Autodesk Inventor part; units mm, degrees
ref_plane "YZ Plane" through (0, 0, 0) normal (1, 0, 0) x (0, 1, 0)
ref_plane "XZ Plane" through (0, 0, 0) normal (0, 1, 0) x (-1, 0, 0)
ref_plane "XY Plane" through (0, 0, 0) normal (0, 0, 1) x (1, 0, 0)
sketch "Sketch1" plane through (0, 0, 0) normal (0, 1, 0) x (-1, 0, 0)
  line L0 (0, 0) -> (28.575, 0)
  line L1 (28.575, 0) -> (0, 0)
  line L2 (0, 0) -> (-14.2875, -24.7467)
  line L3 (0, 0) -> (28.575, 0) construction
  line L4 (0, 0) -> (-14.2875, 24.7467)
  line L5 (0, 0) -> (28.575, 0) construction
  circle A0 centre (28.575, 0) radius 2.54
  circle A1 centre (-14.2875, -24.7467) radius 2.54
  circle A2 centre (-14.2875, 24.7467) radius 2.54
  circle A3 centre (0, 0) radius 3.175
  circle A4 centre (0, 0) radius 6.35
  line L6 (-1.5875, -2.7496) -> (0, 0)
  line L7 (0, 0) -> (-6.35, 0)
  circle A5 centre (-14.2875, 24.7467) radius 3.81
  circle A6 centre (28.575, 0) radius 3.81
  circle A7 centre (-14.2875, -24.7467) radius 3.81
  line L8 (30.6811, 3.175) -> (-12.1814, 27.9217)
  line L9 (28.2054, -3.792) -> (-10.8187, -26.3226)
  line L10 (-18.0975, 24.7467) -> (-18.0975, -24.7467)
  line L11 (0, 0) -> (5.0525, -8.8146)
  line L12 (0, 0) -> (5.1463, 8.7602)
  line L13 (0, 0) -> (-10.16, 0)
  arc A8 (28.2054, -3.792) -> (-10.8187, -26.3226) centre (24.4473, -42.344) ccw
  arc A9 (-10.8187, 26.3226) -> (28.2054, 3.792) centre (24.4473, 42.344) ccw
  arc A10 (-17.3867, -22.5305) -> (-17.3867, 22.5305) centre (-48.8947, 0) ccw
  point P0 (5.1074, 8.7829)
  point P1 (-10.16, 0.0317)
  point P2 (30.2716, 3.4114)
  point P3 (28.2054, 3.792)
  point P4 (-10.8187, 26.3226)
  point P5 (-17.3867, 22.5305)
  point P6 (-17.3867, -22.5305)
  dimension "d9" = 6.35
  dimension "d41" = 12.7
  dimension "d0" = 28.575
  dimension "d1" = 28.575
  dimension "d2" = 120
  dimension "d3" = 28.575
  dimension "d4" = 120
  dimension "d5" = 5.08
  dimension "d6" = 5.08
  dimension "d7" = 5.08
  dimension "d42" = 7.62
  dimension "d43" = 7.62
  dimension "d44" = 7.62
  dimension "d47" = 10.16
  dimension "d48" = 10.16
  dimension "d49" = 10.16
  dimension "d52" = 360
extrude "Extrusion4" add sketch "Sketch1" along normal blind 12.7 contours A3 L12 A4 L0 | L0 A4 L11 A3 | A3 L11 A4 L2 | L2 A4 L7 A3 | A3 L7 A4 L4 | L4 A4 L12 A3 | A4 L12 A9 A6 L0 | L0 A6 A8 L11 A4 | A4 L11 A8 A7 L2 | L2 A7 A10 L13 A4 | A4 L13 A10 A5 L4 | L4 A5 A9 L12 A4 | A6 L8 | A7 | A5 picked at (31.8987, 0.5122)
sketch "Sketch11" plane through (0, 12.7, 0) normal (0, 1, 0) x (1, 0, 0)
  arc A0 (10.8187, -26.3226) -> (-28.2054, -3.792) centre (-24.4473, -42.344) ccw
  arc A1 (17.3867, 22.5305) -> (17.3867, -22.5305) centre (48.8947, 0) ccw
  arc A2 (10.8187, -26.3226) -> (17.3867, -22.5305) centre (14.2875, -24.7467) ccw
  line L0 (0, 0) -> (14.2875, -24.7467)
  circle A3 centre (14.2875, -24.7467) radius 2.54
  line L1 (14.2875, -24.7467) -> (8.2579, -14.3032)
  line L2 (14.2875, -24.7467) -> (7.9375, -13.7482)
  line L3 (7.9375, -13.7482) -> (11.895, -11.4633)
  line L4 (7.9375, -13.7482) -> (3.98, -16.033)
  circle A4 centre (14.2875, 24.7467) radius 2.54
  line L5 (0, 0) -> (14.2875, 24.7467)
  line L6 (14.2875, 24.7467) -> (7.9375, 13.7482)
  line L7 (7.9375, 13.7482) -> (0, 0)
  circle A5 centre (-28.575, 0) radius 2.54
  line L8 (0, 0) -> (-28.575, 0)
  line L9 (-28.575, 0) -> (-15.875, 0)
  line L10 (-15.875, 0) -> (-15.875, 4.5698)
  arc A6 (-28.2054, 3.792) -> (10.8187, 26.3226) centre (-24.4473, 42.344) ccw
  line L11 (-15.875, 0) -> (-15.875, -4.5698)
  line L12 (7.9375, 13.7482) -> (3.98, 16.033)
  line L13 (7.9375, 13.7482) -> (11.895, 11.4633)
  arc A7 (17.3867, 22.5305) -> (17.3867, -22.5305) centre (48.8947, 0) ccw
  arc A8 (-28.2054, 3.792) -> (-30.6811, -3.175) centre (-28.575, 0) ccw
  arc A9 (10.8187, -26.3226) -> (-28.2054, -3.792) centre (-24.4473, -42.344) ccw
  arc A10 (-30.2716, -3.4114) -> (-28.2054, -3.792) centre (-28.575, 0) ccw
  line L14 (-30.6811, -3.175) -> (-30.2716, -3.4114)
  arc A11 (17.3867, 22.5305) -> (10.8187, 26.3226) centre (14.2875, 24.7467) ccw
  point P0 (2.3124, -14.3387)
  point P1 (11.3663, -9.5918)
  point P2 (10.2682, -2.8934)
  point P3 (-3.012, -10.0809)
  dimension "d65" = 12.7
  dimension "d66" = 12.7
  dimension "d67" = 12.7
extrude "Extrusion6" cut sketch "Sketch11" against normal blind 25.4 contours A0 L4 L3 A1 A2 | A0 A10 L14 A8 A6 L10 L11 | L13 L12 A6 A11 A1
sketch "Sketch12" plane through (-15.875, 12.7, -4.5698) normal (-1, 0, 0) x (0, 0, 1)
  line L0 (0, -12.7) -> (0, 0)
  line L1 (0, -6.35) -> (9.0387, -6.35)
  line L2 (1.3948, 0) -> (7.7448, 0)
  line L3 (4.5698, 0) -> (4.5698, -12.7)
  line L4 (9.1395, -12.7) -> (20.6028, -12.7)
  line L5 (9.1395, 0) -> (20.6028, 0)
  line L6 (9.1395, -12.7) -> (9.1395, 0)
  line L7 (9.0387, -6.35) -> (9.1395, -6.35)
  line L8 (9.1395, 0) -> (9.1395, -12.7)
  point P0 (4.5698, -6.35)
sketch "Sketch13" plane through (11.895, 0, 11.4633) normal (0.5, 0, 0.8660254) x (0.8660254, 0, -0.5)
  line L0 (0, 12.7) -> (0, 0)
  line L1 (0, 6.35) -> (-9.1395, 6.35)
  line L2 (-9.1395, 0) -> (-9.1395, 12.7)
  line L3 (-9.1395, 12.7) -> (0, 12.7)
  line L4 (-4.5698, 12.7) -> (-4.5698, 0)
  point P0 (-4.5698, 6.35)
sketch "Sketch14" plane through (3.98, 0, -16.033) normal (0.5, 0, -0.8660254) x (-0.8660254, 0, -0.5)
  line L0 (-9.1395, 0) -> (-9.1395, 12.7)
  line L1 (-9.1395, 6.35) -> (0, 6.35)
  line L2 (0, 12.7) -> (0, 0)
  line L3 (-9.1395, 12.7) -> (0, 12.7)
  line L4 (-4.5698, 12.7) -> (-4.5698, 0)
  point P0 (-4.5698, 6.35)
hole "Hole5" at (7.9375, 6.35, 13.7482) direction (-0.5, 0, -0.8660254) diameter 1.6942 depth 6.6294
hole "Hole6" at (-15.875, 6.35, 0) direction (1, 0, 0) diameter 1.6942 depth 6.6294
hole "Hole7" at (7.9375, 6.35, -13.7482) direction (-0.5, 0, 0.8660254) diameter 1.6942 depth 6.6294
properties part number "stability"
Verification items for the finished model (mm, model axes). A direction names the side the tool comes from. Coordinates: 2 decimals unless noted, no trailing zeros. Write each loop counter-clockwise with the first axis right and the second up, starting at its lowest first coordinate (ties: lowest second). Pieces come first, ordered by that corner, then holes. Notation, with made-up numbers: M -29.75,23 L -16.75,23 A24 ccw -16.75,51 Z; hole C 50.5,86.25 d9. An arc over 180 degrees is marked long. One line per question, with ' | ' between items.
1) Sectioned sample at B-B on x = -10. Record the cut outline in (y, z).
Solutions:
outline: M 0,-6.4 L 12.7,-6.4 L 12.7,6.4 L 0,6.4 Z; hole C 6.35,0 d1.69
2) Material ranges on L1, parallel to Y at x = -11.5, z = 0; L2, parallel to Z at x = 1, y = 11.25; L3, parallel to X at y = 6, z = -8.5, recorded low to high.
Solutions:
L1: 0 to 5.5, 7.2 to 12.7 | L2: -13.14 to -3.01, 3.01 to 13.14 | L3: -5.61 to 4.02, 5.8 to 11.1
3) Sectioned sample at C-C on z = 7. Record the cut outline in (x, y), then the cut area to 3 significant figures.
Solutions:
outline: M -8.6,0 L 10.8,0 L 10.8,12.7 L -8.6,12.7 Z | area: 246 mm^2
4) Release check for a two-part mould opening along X. For faces 1 (the face through (-12.51, 5.51, -0.11)), 2 (the face through (6.538, 7.133, -10.675)), 3 (the face through (-15.875, 6, -1)) record: +X half, -X half, draft (parallel to the pull), parting line (faces both ways), or undercut.
Solutions:
face 1: draft | face 2: undercut | face 3: -X half
5) Depth check by flat-ended pin: pin 1 Ø1.5 at (x, y) = (-8.5, 6) entering from +Z; pin 2 Ø1 at (y, z) = (6.35, 0) entering from +X; pin 3 Ø3 at (x, y) = (7, 11) entering from -Z. Enter the tip coordinate at first touch or a pass-through.
Solutions:
pin 1: z = 7.39 | pin 2: x = 10.16 | pin 3: z = -15.16
6) Access from +Z, -Z, +X, -X, +Y, -Y to the whole of each face (thin tool, end or side, straight path). Record for faces 4 (the face through (4.613, 6.362, 8.013)), 5 (the face through (-9.246, 6, 0)).
Solutions:
face 4: none | face 5: -X
7) Sectioned sample at D-D on y = 6.35. Record the cut outline in (x, z) (3 decimals), then the cut area to 3 significant figures.
Solutions:
outline: M -15.875,-4.57 A38.735 cw 3.98,-16.033 L 7.204,-14.172 L 3.889,-8.431 L 5.356,-7.583 L 8.671,-13.325 L 11.895,-11.463 A38.735 cw 11.895,11.463 L 8.671,13.325 L 5.356,7.583 L 3.889,8.431 L 7.204,14.172 L 3.98,16.033 A38.735 cw -15.875,4.57 L -15.875,0.847 L -9.246,0.847 L -9.246,-0.847 L -15.875,-0.847 Z; hole C 0,0 d6.35 | area: 481 mm^2
